Geometry check sheet. Reference: the model listing, model coordinates, mm. Coordinates: 2 decimals unless noted, no trailing zeros. Loops run counter-clockwise (first coordinate to the right, second up) from the corner with the lowest first, then second, coordinate; pieces in that order, holes last.
from build123d import *

# Parameters (mm, degrees)
SKETCH1_R           = 3.1
BOSS_EXTRUDE1_DEPTH = 6.35
FILLET1_R           = 4


with BuildPart() as part:
    # Sketch1 → Boss-Extrude1 (new body)
    with BuildSketch(Plane(origin=(0, 0, 0), x_dir=(1, 0, 0), z_dir=(0, 1, 0))):
        Polygon((0, -12.7), (-38.1, -12.7), (-38.1, 12.7), (-12.7, 63.5), (12.7, 63.5), (38.1, 12.7), (38.1, -12.7), align=None)
        with Locations(Location((0, 50.8, 0), (0, 0, 270))):
            Circle(SKETCH1_R, mode=Mode.SUBTRACT)
        with Locations(Location((0, 25.4, 0), (0, 0, 270))):
            Circle(SKETCH1_R, mode=Mode.SUBTRACT)
        with Locations(Location((25.4, 0, 0), (0, 0, 270))):
            Circle(SKETCH1_R, mode=Mode.SUBTRACT)
        with Locations(Location((0, 0, 0), (0, 0, 270))):
            Circle(SKETCH1_R, mode=Mode.SUBTRACT)
        with Locations(Location((-25.4, 0, 0), (0, 0, 270))):
            Circle(SKETCH1_R, mode=Mode.SUBTRACT)
    extrude(amount=BOSS_EXTRUDE1_DEPTH)

    # Fillet1
    fillet1_edges = [part.edges().sort_by_distance(p)[0] for p in [
        (-38.1, 3.175, 12.7),
        (-38.1, 3.175, -12.7),
        (-12.7, 3.175, -63.5),
        (12.7, 3.175, -63.5),
        (38.1, 3.175, -12.7),
        (38.1, 3.175, 12.7),
    ]]
    fillet(fillet1_edges, radius=FILLET1_R)


solid = part.part
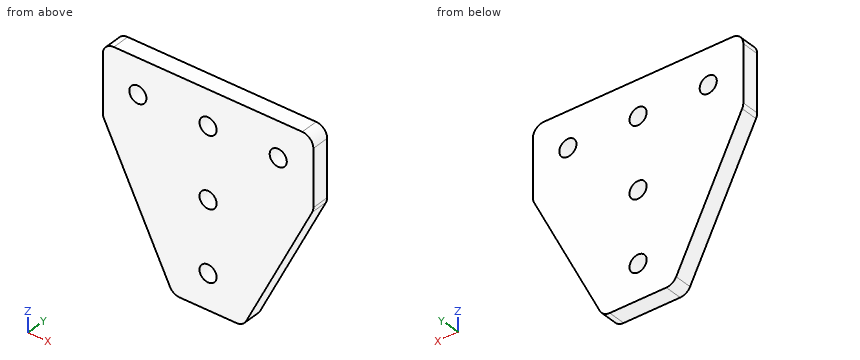
(1) Sectioned sample at A-A on x = 25.4. Record the cut outline in (y, z).
Findings:
outline: (0, -38.1) - (6.35, -38.1) - (6.35, -3.1) - (0, -3.1) - close; (0, 3.1) - (6.35, 3.1) - (6.35, 12.7) - (0, 12.7) - close
(2) Sectioned sample at C-C on y = 4.5. Record the cut outline in (x, z).
Findings:
outline: (-38.1, -11.76) arc R4 ccw to (-37.68, -13.54) - (-13.81, -61.29) arc R4 ccw to (-10.23, -63.5) - (10.23, -63.5) arc R4 ccw to (13.81, -61.29) - (37.68, -13.54) arc R4 ccw to (38.1, -11.76) - (38.1, 8.7) arc R4 ccw to (34.1, 12.7) - (-34.1, 12.7) arc R4 ccw to (-38.1, 8.7) - close; hole circle Ø6.2 at (-25.4, 0); hole circle Ø6.2 at (0, -50.8); hole circle Ø6.2 at (0, -25.4); hole circle Ø6.2 at (0, 0); hole circle Ø6.2 at (25.4, 0)
(3) Sectioned sample at B-B on z = 0. Record the cut outline in (x, y), and give its area (3 significant figures).
Findings:
outline: (-38.1, 0) - (-28.5, 0) - (-28.5, 6.35) - (-38.1, 6.35) - close; (-22.3, 0) - (-3.1, 0) - (-3.1, 6.35) - (-22.3, 6.35) - close; (3.1, 0) - (22.3, 0) - (22.3, 6.35) - (3.1, 6.35) - close; (28.5, 0) - (38.1, 0) - (38.1, 6.35) - (28.5, 6.35) - close
area: 366 mm2
(4) Sectioned sample at D-D on z = -42.5. Record the cut outline in (x, y), and give its area (3 significant figures).
Findings:
outline: (-23.2, 0) - (23.2, 0) - (23.2, 6.35) - (-23.2, 6.35) - close
area: 295 mm2
(5) Scan lines: L1, parallel to X at y = 1.75, z = 0; L2, parallel to Z at x = 23, y = 5.75; L3, parallel to Z at x = 26.5, y = 5.25. Record each from-to range of solid material in increasing order.
Findings:
L1: x = -38.1 to -28.5, -22.3 to -3.1, 3.1 to 22.3, 28.5 to 38.1
L2: z = -42.9 to -1.96, 1.96 to 12.7
L3: z = -35.9 to -2.9, 2.9 to 12.7
(6) Gauge pin test, flat ends, axial feed: pin 1 Ø8 at (x, z) = (0, -50.8) entering from +Y; pin 2 Ø2 at (y, z) = (4, -51.5) entering from +X; pin 3 Ø5.5 at (x, z) = (0, 0) entering from +Y. Record the tip position at first contact, or that the pin passes through.
Findings:
pin 1: stops at y = 6.35
pin 2: stops at x = 19.2
pin 3: passes through
